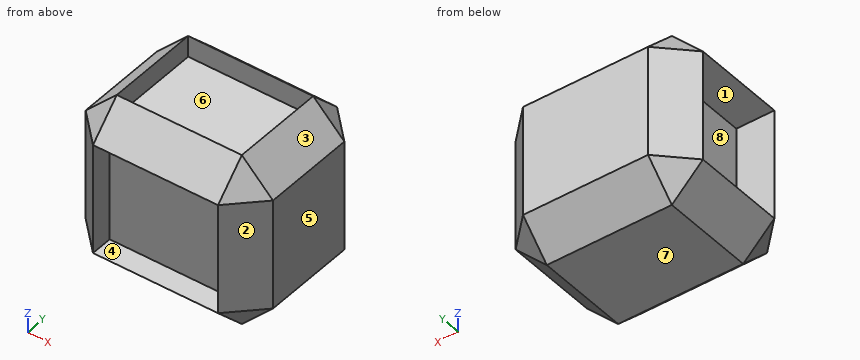
from build123d import *

# Parameters (mm, degrees)
F0_W     = 30.0513710827
F0_H     = 27.739726007
F1_DEPTH = 25
F2_SIZE  = 5
F3_DEPTH = 6.1
F4_DEPTH = 3.4
F5_DEPTH = 3.5


with BuildPart() as f1:
    # F0 (on Front) → F1 (new body)
    with BuildSketch(Plane.XZ):
        with Locations((-15.0256855413, 13.8698630035)):
            Rectangle(F0_W, F0_H)
    extrude(amount=F1_DEPTH)

    # F2
    f2_edges = [f1.edges().sort_by_distance(p)[0] for p in [
        (-15.025686, -25, 27.739726),
        (0, -25, 13.869863),
        (-15.025686, -25, 0),
        (-30.051371, -25, 13.869863),
        (-30.051371, -12.5, 27.739726),
        (0, -12.5, 27.739726),
        (-15.025686, 0, 27.739726),
        (0, 0, 13.869863),
        (-30.051371, 0, 13.869863),
        (-30.051371, -12.5, 0),
        (-15.025686, 0, 0),
        (0, -12.5, 0),
    ]]
    chamfer(f2_edges, length=F2_SIZE)

    # F3 (cut): a face of the model
    f3_faces = [f1.faces().sort_by_distance(p)[0] for p in [
        (-30.0513710827, -12.5, 13.8698630035),
    ]]
    extrude(f3_faces, amount=-F3_DEPTH, mode=Mode.SUBTRACT)

    # F4 (cut): a face of the model
    f4_faces = [f1.faces().sort_by_distance(p)[0] for p in [
        (-15.0256855413, -12.5, 27.739726007),
    ]]
    extrude(f4_faces, amount=-F4_DEPTH, mode=Mode.SUBTRACT)

    # F5 (cut): a face of the model
    f5_faces = [f1.faces().sort_by_distance(p)[0] for p in [
        (-15.0256855413, -25, 13.8698630035),
    ]]
    extrude(f5_faces, amount=-F5_DEPTH, mode=Mode.SUBTRACT)


solid = f1.part
Verification items for the finished model (mm, model axes). Face numbers are marked on the shaded views. A direction names the side the tool comes from. Give positions to 0.01 mm unless a question says otherwise; leave off trailing zeros. Order: outer loops, then holes, each group sorted by start corner. A loop starts at its lowest first (then second) coordinate and runs counter-clockwise, first axis right, second up. Notation, with made-up numbers: (-26.5, 72) -> (30.5, 72) arc R19 ccw to (30.5, 87) -> close; hole circle Ø7 at (-39.5, 10.5). An arc over 180 degrees is marked (long way). Answer as CSV lines item,"result".
Q1. Sectioned sample at B-B on y = -7. Record the cut outline in (x, z), plus the area to 3 significant figures.
Solutions:
outline,"(-30.05, 5) -> (-25.05, 0) -> (-5, 0) -> (0, 5) -> (0, 22.74) -> (-5, 27.74) -> (-5, 24.34) -> (-25.05, 24.34) -> (-25.05, 27.74) -> (-30.05, 22.74) -> (-23.95, 22.74) -> (-23.95, 5) -> close"
area,"607 mm²"
Q2. Scan lines: probe 1 along Z at (x, y) = (-24, -5.25); probe 2 along Y at (x, z) = (-20, 19.5); probe 3 along Z at (x, y) = (-20, -8.25). Record each from-to range of solid material in increasing order.
Solutions:
probe 1,"z = 0 to 5, 22.74 to 24.34"
probe 2,"y = -21.5 to 0"
probe 3,"z = 0 to 24.34"
Q3. Sectioned sample at C-C on z = 23.5. Record the cut outline in (x, y), plus the area to 3 significant figures.
Solutions:
outline,"(-29.29, -20) -> (-25.05, -24.24) -> (-5, -24.24) -> (-0.76, -20) -> (-0.76, -5) -> (-5, -0.76) -> (-25.05, -0.76) -> (-29.29, -5) -> close"
area,"634 mm²"
Q4. Depth check by flat-ended pin: pin 1 (3 mm diameter, centred on x = -26.5, z = 13, fed in from -Y); pin 2 (3 mm diameter, centred on x = -27, y = -14, fed in from +Z); pin 3 (3 mm diameter, centred on y = -22.5, z = 16.5, fed in from -X). Enter the tip coordinate at first touch or a pass-through.
Solutions:
pin 1,"stops at y = -25"
pin 2,"stops at z = 27.29"
pin 3,"stops at x = -29.05"
Q5. Access from +Z, -Z, +X, -X, +Y, -Y to the whole of each face (thin tool, end or side, straight path). Record for the marked faces 4, 5, 6, 7 and 8.
Solutions:
face 4,"-Y"
face 5,"+Z, -Z, +X, +Y, -Y"
face 6,"+Z"
face 7,"-Z, +X, -X, +Y, -Y"
face 8,"-X"
Q6. Sectioned sample at D-D on x = -28. Record the cut outline in (y, z).
Solutions:
outline,"(-22.05, 5) -> (-20, 2.95) -> (-5, 2.95) -> (-2.95, 5) -> (-2.95, 22.74) -> (-5, 24.79) -> (-20, 24.79) -> (-22.05, 22.74) -> close; hole (-20, 5) -> (-5, 5) -> (-5, 22.74) -> (-20, 22.74) -> close"
Q7. Release check for a two-part mould opening along Y. For the marked faces 1, 2 and 3 record: +Y half, -Y half, draft (parallel to the pull), parting line (faces both ways), or undercut.
Solutions:
face 1,"undercut"
face 2,"-Y half"
face 3,"draft"
Q8. Sectioned sample at A-A on x = -22.5. Record the cut outline in (y, z).
Solutions:
outline,"(-25, 5) -> (-20, 0) -> (-5, 0) -> (0, 5) -> (0, 22.74) -> (-5, 27.74) -> (-5, 24.34) -> (-20, 24.34) -> (-20, 27.74) -> (-25, 22.74) -> (-21.5, 22.74) -> (-21.5, 5) -> close"
